Source: CAD feature listing. Evaluate the final solid. Frame: model axes, mm. A direction names the side the tool comes from. Coordinates: 2 decimals unless noted, no trailing zeros. Write each loop counter-clockwise with the first axis right and the second up, starting at its lowest first coordinate (ties: lowest second). Pieces come first, ordered by that corner, then holes. Notation, with made-up numbers: M 13.25,67 L 54.25,67 A19 ccw 54.25,99 Z; hole C 63,-25 d2. An arc over 180 degrees is marked long. Write item = value, one per line. Start each with the question number.
1. Access query for faces 1 (the face through (-168.54, 27, 0)), 2 (the face through (-39.731, 23.523, 44.442)), 3 (the face through (48.657, 23.523, 43.946)). Directions: +Z, -Z, +X, -X, +Y, -Y. A direction counts if a zero-diameter tool reaches every point of the face in a straight line with its end or side. Return the directions, or none.
2. Section query B-B (y = 62). Output: boundary loops of the cut face in (x, z), then the cut area to 3 significant figures.
3. Pin query (flat end, axial travel): pin 1 Ø3 at (x, y) = (-74, 47.5) entering from +Z; pin 2 Ø2 at (x, y) = (16, 54.5) entering from +Z; pin 3 Ø1.5 at (y, z) = (15.5, 27) entering from -X. Return the tip coordinate at first contact, or that it passes through.
4. Section query C-C (x = -94.5). Output: boundary loops of the cut face in (y, z), then the cut area to 3 significant figures.
5. Pull-direction query (Z, two-part tool) for faces 4 (the face through (59.16, 4.44, -54.31)), 5 (the face through (-104, 48.47, -26.46)), 6 (the face through (-121, 46.5, -1)), 7 (the face through (-46, 0, -1)); classes: pulls with the +Z half, pulls with the -Z half, needs draft (parallel to the pull), parting line crosses it, or undercut.
6. Line query: line 1 along X through (y, z) = (27.5, 6); line 2 along Y through (x, z) = (-41, 20); line 3 along Y through (x, z) = (-123.5, -44.5). Output: solid intervals per line, ascending.
7. Section query A-A (x = -143). Output: boundary loops of the cut face in (y, z).
```python
from build123d import *

# Parameters (mm, degrees)
EXTRUDE_1_DEPTH     = 9
CUT_EXTRUDE_2_DEPTH = 9
SKETCH_4_R          = 63.5
EXTRUDE_2_DEPTH     = 60
EXTRUDE_3_DEPTH     = 37.5
EXTRUDE_4_DEPTH     = 4
EXTRUDE_5_DEPTH     = 25
EXTRUDE_6_DEPTH     = 25
EXTRUDE_7_DEPTH     = 25
CUT_EXTRUDE2_START  = -60
SKETCH4_R           = 63.5
SKETCH4_R_2         = 62.5
CUT_EXTRUDE2_DEPTH  = 60
CUT_EXTRUDE4_DEPTH  = 6.8
CIRPATTERN1_COUNT   = 8
SKETCH15_W          = 73.49693164
SKETCH15_H          = 33.050154469
BOSS_EXTRUDE4_DEPTH = 16
SKETCH16_W          = 25
SKETCH16_H          = 20
BOSS_EXTRUDE5_DEPTH = 10
CUT_EXTRUDE5_DEPTH  = 20
SKETCH19_W          = 10
SKETCH19_H          = 84
CUT_EXTRUDE6_DEPTH  = 41.5


with BuildPart() as part:
    # 草图1 → 凸台-拉伸1 (new body)
    with BuildSketch(Plane(origin=(0, 0, 0), x_dir=(1, 0, 0), z_dir=(0, 1, 0))):
        Polygon((81.469684938, 32), (36.214850942, 77.254833996), (-27.785149058, 77.254833996), (-53.539983054, 51.5), (-170.539983054, 51.5), (-170.539983054, -51.5), (-53.539983054, -51.5), (-27.785149058, -77.254833996), (36.214850942, -77.254833996), (81.469684938, -32), align=None)
    extrude(amount=EXTRUDE_1_DEPTH)

    # 草图2 → 切除-拉伸2 (cut)
    with BuildSketch(Plane(origin=(0, 9, 0), x_dir=(1, 0, 0), z_dir=(0, 1, 0))):
        Polygon((-151.539983054, -51.5), (-170.539983054, -32.5), (-170.539983054, -51.5), align=None)
        Polygon((-170.539983054, 51.5), (-170.539983054, 32.5), (-151.539983054, 51.5), align=None)
    extrude(amount=-CUT_EXTRUDE_2_DEPTH, mode=Mode.SUBTRACT)

    # 草图4 → 凸台-拉伸2 (add)
    with BuildSketch(Plane(origin=(0, 9, 0), x_dir=(1, 0, 0), z_dir=(0, 1, 0))):
        with Locations(Location((4.214850942, 0, 0), (0, 0, 270))):
            Circle(SKETCH_4_R)
    extrude(amount=EXTRUDE_2_DEPTH)

    # 草图5 → 凸台-拉伸3 (add)
    with BuildSketch(Plane(origin=(0, 9, 0), x_dir=(1, 0, 0), z_dir=(0, 1, 0))):
        Polygon((-155.539983054, -42), (-61.539983054, -42), (-61.539983054, 42), (-155.539983054, 42), (-168.539983054, 29), (-168.539983054, -29), align=None)
    extrude(amount=EXTRUDE_3_DEPTH)

    # 草图7 → 凸台-拉伸4 (add)
    with BuildSketch(Plane(origin=(0, 46.5, 0), x_dir=(1, 0, 0), z_dir=(0, 1, 0))):
        Polygon((-106.539983054, 42), (-61.539983054, 42), (-61.539983054, 29), (-66.539983054, 24), (-101.539983054, 24), (-106.539983054, 29), align=None)
        Polygon((-106.539983054, -29), (-101.557170407, -24), (-66.5227957, -24), (-61.539983054, -29), (-61.539983054, -42), (-106.539983054, -42), align=None)
    extrude(amount=EXTRUDE_4_DEPTH)

    # 草图8 → 凸台-拉伸5 (add)
    with BuildSketch(Plane.ZY.offset(101.539983054)):
        Polygon((-24, 46.5), (-10, 66.5), (10, 66.5), (24, 46.5), (24, 89.5), (20, 89.5), (10, 79), (10, 75), (-10, 75), (-10, 79), (-20, 89.5), (-24, 89.5), align=None)
    extrude(amount=-EXTRUDE_5_DEPTH)

    # 草图12 → 凸台-拉伸6 (add)
    with BuildSketch(Plane.ZY.offset(101.539983054)):
        Polygon((-24, 58.5), (-27, 50.5), (-24, 50.5), align=None)
    extrude(amount=-EXTRUDE_6_DEPTH)

    # 草图15 → 凸台-拉伸7 (add)
    with BuildSketch(Plane.ZY.offset(101.539983054)):
        Polygon((24, 50.5), (27, 50.5), (24, 58.5), align=None)
    extrude(amount=-EXTRUDE_7_DEPTH)

    # Sketch4 → Cut-Extrude2 (cut)
    with BuildSketch(Plane(origin=(0, 69, 0), x_dir=(1, 0, 0), z_dir=(0, 1, 0)).offset(CUT_EXTRUDE2_START)):
        with Locations((4.214850942, 0)):
            Circle(SKETCH4_R)
        with Locations(Location((4.214850942, 0, 0), (0, 0, 270))):
            Circle(SKETCH4_R_2, mode=Mode.SUBTRACT)
    extrude(amount=CUT_EXTRUDE2_DEPTH, mode=Mode.SUBTRACT)

    # Sketch9 → Revolve2 (revolve)
    with BuildSketch(Plane.XY, mode=Mode.PRIVATE) as revolve2_sk:
        Polygon((66.714850942, 45.698851706), (71.557167148, 9), (66.714850942, 9), align=None)
    revolve(revolve2_sk.sketch.rotate(Axis((4.214850942, 69, 0), (0, 1, 0)), 167.534637939), axis=Axis((4.214850942, 69, 0), (0, 1, 0)))

    # Sketch12 → Cut-Extrude4 (cut)
    with BuildSketch(Plane.XY.offset(62.5)):
        with BuildLine():
            Line((36.214850942, 9), (-27.785149058, 9))
            add(Edge.make_bspline(
                [(-27.785149058, 9), (-0.604837494, 82.63399563), (36.214850942, 9)],
                knots=[0, 0, 0, 1, 1, 1], degree=2))
        make_face()
    cut_extrude4 = extrude(amount=CUT_EXTRUDE4_DEPTH, mode=Mode.SUBTRACT)

    # CirPattern1: Cut-Extrude4 ×8 about axis
    cirpattern1_axis = Axis((4.214850942, 69, 0), (0, 1, 0))
    for i in range(1, CIRPATTERN1_COUNT):
        add(cut_extrude4.rotate(cirpattern1_axis, i * 360 / CIRPATTERN1_COUNT), mode=Mode.SUBTRACT)

    # Sketch15 → Boss-Extrude4 (add)
    with BuildSketch(Plane(origin=(-61.539983054, 0, 0), x_dir=(0, 0, -1), z_dir=(1, 0, 0))):
        with Locations((3.027242224, 22.608056987)):
            Rectangle(SKETCH15_W, SKETCH15_H)
    extrude(amount=-BOSS_EXTRUDE4_DEPTH)

    # Sketch16 → Boss-Extrude5 (add)
    with BuildSketch(Plane(origin=(0, 75, 0), x_dir=(1, 0, 0), z_dir=(0, 1, 0))):
        with Locations((-89.039983054, 0)):
            Rectangle(SKETCH16_W, SKETCH16_H)
    extrude(amount=BOSS_EXTRUDE5_DEPTH)

    # Sketch17 → Cut-Extrude5 (cut)
    with BuildSketch(Plane.XY.offset(10)):
        Polygon((-76.539983054, 79), (-101.539983054, 71.348105906), (-101.539983054, 89.5), (-76.539983054, 89.5), align=None)
    extrude(amount=-CUT_EXTRUDE5_DEPTH, mode=Mode.SUBTRACT)

    # Sketch19 → Cut-Extrude6 (cut)
    with BuildSketch(Plane(origin=(0, 50.5, 0), x_dir=(1, 0, 0), z_dir=(0, 1, 0))):
        with Locations((-66.539983054, 0)):
            Rectangle(SKETCH19_W, SKETCH19_H)
    extrude(amount=-CUT_EXTRUDE6_DEPTH, mode=Mode.SUBTRACT)


solid = part.part
```
Results are:
q1.face_1 = +Z, -Z, -X, +Y
q1.face_2 = +Z, +Y
q1.face_3 = +Z, +X, +Y
q2.outline = M -101.54,-24 L -76.54,-24 L -76.54,-13.15 L -101.54,-13.15 Z; M -101.54,13.15 L -76.54,13.15 L -76.54,24 L -101.54,24 Z; C 4.21,0 d125
q2.area = 12,800 mm^2
q3.pin_1 = 42
q3.pin_2 = 61.56
q3.pin_3 = -168.54
q4.outline = M 0,-51.5 L 9,-51.5 L 9,-42 L 50.5,-42 L 50.5,-27 L 58.5,-24 L 89.5,-24 L 89.5,-20 L 79,-10 L 73.5,-10 L 73.5,10 L 79,10 L 89.5,20 L 89.5,24 L 58.5,24 L 50.5,27 L 50.5,42 L 9,42 L 9,51.5 L 0,51.5 Z; hole M 46.5,-24 L 66.5,-10 L 66.5,10 L 46.5,24 Z
q4.area = 5,200 mm^2
q5.face_4 = pulls with the -Z half
q5.face_5 = undercut
q5.face_6 = undercut
q5.face_7 = needs draft
q6.line_1 = -168.54 to -71.54, -58.29 to 66.71
q6.line_2 = 0 to 69
q6.line_3 = 0 to 9
q7.outline = M 0,-51.5 L 9,-51.5 L 9,-42 L 46.5,-42 L 46.5,42 L 9,42 L 9,51.5 L 0,51.5 Z
